Geometry check sheet. Reference: the model listing, model coordinates, mm. A direction names the side the tool comes from. Give positions to 0.01 mm unless a question says otherwise; leave off trailing zeros. Order: outer loops, then holes, each group sorted by start corner. A loop starts at its lowest first (then second) coordinate and runs counter-clockwise, first axis right, second up. Notation, with made-up numbers: M 22,-25 L 69,-25 A21 ccw 69,-9 Z; hole C 2,75 d3. An arc over 180 degrees is marked long. One line per question, with ' | ' between items. Start each with the question number.
from build123d import *

# Parameters (mm, degrees)
SKETCH1_W           = 539
SKETCH1_H           = 299
BOSS_EXTRUDE1_DEPTH = 1.5
SKETCH10_W          = 70
SKETCH10_H          = 20
CUT_EXTRUDE6_DEPTH  = 309.192715683
SKETCH2_R           = 3
SKETCH2_R_2         = 2
CUT_EXTRUDE1_DEPTH  = 10
CUT_EXTRUDE7_DEPTH  = 309.192715683


with BuildPart() as part:
    # Sketch1 → Boss-Extrude1 (new body)
    with BuildSketch(Plane(origin=(0, 0, 0), x_dir=(1, 0, 0), z_dir=(0, 1, 0))):
        Rectangle(SKETCH1_W, SKETCH1_H)
    extrude(amount=-BOSS_EXTRUDE1_DEPTH)

    # Sketch10 → Cut-Extrude6 (cut, through all)
    with BuildSketch(Plane(origin=(0, 0, 0), x_dir=(1, 0, 0), z_dir=(0, 1, 0))):
        Polygon((269.5, 149.5), (199.5, 149.5), (199.5, 129.5), (249.5, 129.5), (249.5, 91.5), (269.5, 91.5), align=None)
        with Locations((234.5, -139.5)):
            Rectangle(SKETCH10_W, SKETCH10_H)
    extrude(amount=-CUT_EXTRUDE6_DEPTH, mode=Mode.SUBTRACT)

    # Sketch2 → Cut-Extrude1 (cut)
    with BuildSketch(Plane(origin=(0, 0, 0), x_dir=(1, 0, 0), z_dir=(0, 1, 0))):
        with Locations(Location((-260, 0, 0), (0, 0, 270))):
            Circle(SKETCH2_R)
        with Locations(Location((-260, 15, 0), (0, 0, 270))):
            Circle(SKETCH2_R_2)
        with Locations(Location((-260, -15, 0), (0, 0, 270))):
            Circle(SKETCH2_R_2)
    cut_extrude1 = extrude(amount=-CUT_EXTRUDE1_DEPTH, mode=Mode.SUBTRACT)

    # Mirror1: Cut-Extrude1 across plane
    add(cut_extrude1.mirror(Plane(origin=(0, 0, 0), x_dir=(0, 0, 1), z_dir=(1, 0, 0))), mode=Mode.SUBTRACT)

    # Sketch11 → Cut-Extrude7 (cut, through all)
    with BuildSketch(Plane(origin=(0, 0, 0), x_dir=(1, 0, 0), z_dir=(0, 1, 0))):
        Polygon((227.025012956, 3), (227.025012956, -3), (100, -30), (90.5, -30), (90.5, -40), (69.5, -40), (69.5, -30), (50.5, -30), (50.5, -40), (29.5, -40), (29.5, -30), (10.5, -30), (10.5, -45), (-10.5, -45), (-10.5, -30), (-29.5, -30), (-29.5, -40), (-50.5, -40), (-50.5, -30), (-69.5, -30), (-69.5, -40), (-90.5, -40), (-90.5, -30), (-100, -30), (-227.025012956, -3), (-227.025012956, 3), (-100, 30), (-90.5, 30), (-90.5, 40), (-69.5, 40), (-69.5, 30), (-50.5, 30), (-50.5, 40), (-29.5, 40), (-29.5, 30), (-10.5, 30), (-10.5, 45), (10.5, 45), (10.5, 30), (29.5, 30), (29.5, 40), (50.5, 40), (50.5, 30), (69.5, 30), (69.5, 40), (90.5, 40), (90.5, 30), (100, 30), align=None)
    extrude(amount=-CUT_EXTRUDE7_DEPTH, mode=Mode.SUBTRACT)


solid = part.part
Item 1: Mould release check, pull along Z, two halves, no side actions. Record for faces 1 (the flat face through (-64, -1.5, -35)), 2 (the flat face through (162.62, -0.74, -16.69)): released by +Z, released by -Z, zero draft, split by the parting line, or undercut.
Item 2: Cross-section at A-A, the plane x = -84. Record the cut outline in (y, z), plus the area to 4 significant figures.
Item 3: Material ranges on line 1 along Z through (x, y) = (260, -0.4); line 2 along X through (y, z) = (-0.95, 0); line 3 along Z through (x, y) = (-260, -0.7), recorded low to high.
Item 4: Cross-section at C-C, the plane x = 123. Record the cut outline in (y, z), plus the area to 3 significant figures.
Item 5: Cross-section at B-B, the plane y = -1. State how many separate pieces and enclosed holes the cut face has, plus the area to 3 significant figures.
Item 6: Depth check by flat-ended pin: pin 1 (3 mm diameter, centred on x = -154.5, z = 82, fed in from +Y). Enter the tip coordinate at first touch or a pass-through.
Item 7: Set-up check for faces 3 (the flat face through (-64, 0, -35)), 4 (the flat face through (164.4, -0.74, 16.31)): record each of +Z, -Z, +X, -X, +Y, -Y from which the full face is reachable in a straight line by a thin tool's end or side.
Outcome:
1) face 1: zero draft | face 2: undercut
2) outline: M -1.5,-149.5 L 0,-149.5 L 0,-40 L -1.5,-40 Z; M -1.5,40 L 0,40 L 0,149.5 L -1.5,149.5 Z | area: 328.5 mm²
3) line 1: z = -91.5 to -17, -13 to -3, 3 to 13, 17 to 129.5 | line 2: x = -269.5 to -263, -257 to -227.03, 227.03 to 257, 263 to 269.5 | line 3: z = -149.5 to -17, -13 to -3, 3 to 13, 17 to 149.5
4) outline: M -1.5,-149.5 L 0,-149.5 L 0,-25.11 L -1.5,-25.11 Z; M -1.5,25.11 L 0,25.11 L 0,149.5 L -1.5,149.5 Z | area: 373 mm²
5) separate pieces: 1 | enclosed holes: 7 | area: 135,000 mm²
6) pin 1: stops at y = 0
7) face 3: +Z, -Z, +X, -X, +Y | face 4: +Y, -Y
